```python
from build123d import *

# Parameters (mm, degrees)
F0_W     = 82.55
F0_H     = 82.55
F1_DEPTH = 137.9474
F2_R     = 36.5125
F3_DEPTH = 1.5748
F4_R     = 9.525
F5_DEPTH = 38.1


with BuildPart() as f1:
    # F0 (on Front) → F1 (new body)
    with BuildSketch(Plane.XZ):
        Rectangle(F0_W, F0_H)
    extrude(amount=-F1_DEPTH)

    # F2 (on Front) → F3 (join)
    with BuildSketch(Plane.XZ):
        Circle(F2_R)
    extrude(amount=F3_DEPTH)

    # F4 (on Front) → F5 (join)
    with BuildSketch(Plane.XZ):
        Circle(F4_R)
    extrude(amount=F5_DEPTH)


solid = f1.part
```
Build history of the part. All positions in model axes, mm. A direction names the side the tool comes from. Round coordinates to 2 decimals unless told otherwise and drop trailing zeros. Order: outer loops, then holes, each group sorted by start corner. A loop starts at its lowest first (then second) coordinate and runs counter-clockwise, first axis right, second up. Notation, with made-up numbers: (0, -40) - (55, -40) arc R16 cw to (55, -26) - close; hole circle Ø8 at (81, -2.75). An arc over 180 degrees is marked (long way). Use a Markdown table: item, result.
1) Saw through at D-D on x = 11.5. Write the cut outline in (y, z) (3 decimals), and give its area (3 significant figures).
Recorded:
| item | result |
|---|---|
| outline | (-1.575, -34.654) - (0, -34.654) - (0, -41.275) - (137.947, -41.275) - (137.947, 41.275) - (0, 41.275) - (0, 34.654) - (-1.575, 34.654) - close |
| area | 11,500 mm² |
2) Flat gauge pins, fed straight in: pin 1 Ø3 at (y, z) = (-15, 6.5) entering from +X; pin 2 Ø25 at (x, z) = (12.5, -18.5) entering from -Y. Where does each tip first touch, or does it go through?
Recorded:
| item | result |
|---|---|
| pin 1 | stops at x = 8.11 |
| pin 2 | stops at y = -1.57 |
3) Tool access for faces 1 (the face through (-37, 0, 1)), 2 (the face through (-1, 68, 41.275)): list every direction of +Z, -Z, +X, -X, +Y, -Y with a clear straight run to the whole face (end or side of a thin tool).
Recorded:
| item | result |
|---|---|
| face 1 | -Y |
| face 2 | +Z, +X, -X, +Y, -Y |
4) Wall check: L1, parallel to Y at x = -6.5, z = 8.5; L2, parallel to Y at x = 38.5, z = 38; L3, parallel to Z at x = 11.5, y = -1. Give the ranges that are in metal, low to high.
Recorded:
| item | result |
|---|---|
| L1 | y = -1.57 to 137.95 |
| L2 | y = 0 to 137.95 |
| L3 | z = -34.65 to 34.65 |
5) Saw through at B-B on x = 0. Write the cut outline in (y, z) (1 decimal), and give its area (3 significant figures).
Recorded:
| item | result |
|---|---|
| outline | (-38.1, -9.5) - (-1.6, -9.5) - (-1.6, -36.5) - (0, -36.5) - (0, -41.3) - (137.9, -41.3) - (137.9, 41.3) - (0, 41.3) - (0, 36.5) - (-1.6, 36.5) - (-1.6, 9.5) - (-38.1, 9.5) - close |
| area | 12,200 mm² |
6) Saw through at C-C on z = 24. Write the cut outline in (x, y) (3 decimals).
Recorded:
| item | result |
|---|---|
| outline | (-41.275, 0) - (-27.517, 0) - (-27.517, -1.575) - (27.517, -1.575) - (27.517, 0) - (41.275, 0) - (41.275, 137.947) - (-41.275, 137.947) - close |
7) Saw through at A-A on z = 0. Write the cut outline in (x, y) (1 decimal).
Recorded:
| item | result |
|---|---|
| outline | (-41.3, 0) - (-36.5, 0) - (-36.5, -1.6) - (-9.5, -1.6) - (-9.5, -38.1) - (9.5, -38.1) - (9.5, -1.6) - (36.5, -1.6) - (36.5, 0) - (41.3, 0) - (41.3, 137.9) - (-41.3, 137.9) - close |
